Input: part model. Units: mm. Frame: model coordinates. A direction names the side the tool comes from. Give positions to 0.01 mm unless a question says otherwise; leave off trailing zeros. Loops run counter-clockwise (first coordinate to the right, second up) from the corner with the lowest first, then second, coordinate; pieces in that order, holes last. Notation, with made-up numbers: (51.5, 40.5) - (63.5, 40.5) arc R24 ccw to (63.5, 59.5) - close; hole circle Ø9 at (68, 19.25). An arc over 180 degrees is marked (long way). Answer as a JSON object with one key per item and string values.
from build123d import *

# Parameters (mm, degrees)
F0_R     = 3.5
F1_DEPTH = 25
F2_DEPTH = 2
F3_DEPTH = 10
F4_DEPTH = 21


with BuildPart() as f1:
    # F0 (on Top) → F1 (new body)
    with BuildSketch(Plane.XY):
        with BuildLine():
            ThreePointArc((10.25, -7.1545440106), (5, 0), (10.25, 7.1545440106))
            ThreePointArc((10.25, 7.1545440106), (8.8388347648, 8.8388347648), (7.1545440106, 10.25))
            ThreePointArc((7.1545440106, 10.25), (0, 5), (-7.1545440106, 10.25))
            ThreePointArc((-7.1545440106, 10.25), (-8.8388347648, 8.8388347648), (-10.25, 7.1545440106))
            ThreePointArc((-10.25, 7.1545440106), (-6.4533066888, 4.4370598373), (-5, 0))
            ThreePointArc((-5, 0), (-6.4533066888, -4.4370598373), (-10.25, -7.1545440106))
            ThreePointArc((-10.25, -7.1545440106), (-8.8388347648, -8.8388347648), (-7.1545440106, -10.25))
            ThreePointArc((-7.1545440106, -10.25), (0, -5), (7.1545440106, -10.25))
            ThreePointArc((7.1545440106, -10.25), (8.8388347648, -8.8388347648), (10.25, -7.1545440106))
        make_face()
        Circle(F0_R, mode=Mode.SUBTRACT)
        with BuildLine():
            ThreePointArc((-7.1545440106, 10.25), (0, 5), (7.1545440106, 10.25))
            ThreePointArc((7.1545440106, 10.25), (5.3824617408, 11.2818041823), (3.4655302625, 12.01))
            ThreePointArc((3.4655302625, 12.01), (0, 9), (-3.4655302625, 12.01))
            ThreePointArc((-3.4655302625, 12.01), (-5.3824617408, 11.2818041823), (-7.1545440106, 10.25))
        make_face()
        with BuildLine():
            ThreePointArc((-5, 0), (-6.4533066888, 4.4370598373), (-10.25, 7.1545440106))
            ThreePointArc((-10.25, 7.1545440106), (-11.2818041823, 5.3824617408), (-12.01, 3.4655302625))
            ThreePointArc((-12.01, 3.4655302625), (-9.8575579477, 2.2951034835), (-9, 0))
            ThreePointArc((-9, 0), (-9.8575579477, -2.2951034835), (-12.01, -3.4655302625))
            ThreePointArc((-12.01, -3.4655302625), (-11.2818041823, -5.3824617408), (-10.25, -7.1545440106))
            ThreePointArc((-10.25, -7.1545440106), (-6.4533066888, -4.4370598373), (-5, 0))
        make_face()
        with BuildLine():
            ThreePointArc((3.4655302625, -12.01), (5.3824617408, -11.2818041823), (7.1545440106, -10.25))
            ThreePointArc((7.1545440106, -10.25), (0, -5), (-7.1545440106, -10.25))
            ThreePointArc((-7.1545440106, -10.25), (-5.3824617408, -11.2818041823), (-3.4655302625, -12.01))
            ThreePointArc((-3.4655302625, -12.01), (0, -9), (3.4655302625, -12.01))
        make_face()
        with BuildLine():
            ThreePointArc((12.01, -3.4655302625), (9, 0), (12.01, 3.4655302625))
            ThreePointArc((12.01, 3.4655302625), (11.2818041823, 5.3824617408), (10.25, 7.1545440106))
            ThreePointArc((10.25, 7.1545440106), (5, 0), (10.25, -7.1545440106))
            ThreePointArc((10.25, -7.1545440106), (11.2818041823, -5.3824617408), (12.01, -3.4655302625))
        make_face()
        with BuildLine():
            ThreePointArc((10.25, 7.1545440106), (11.2818041823, 5.3824617408), (12.01, 3.4655302625))
            ThreePointArc((12.01, 3.4655302625), (14.7951034835, 2.6424420523), (16, 0))
            ThreePointArc((16, 0), (14.7951034835, -2.6424420523), (12.01, -3.4655302625))
            ThreePointArc((12.01, -3.4655302625), (11.2818041823, -5.3824617408), (10.25, -7.1545440106))
            ThreePointArc((10.25, -7.1545440106), (16.9370598373, -6.0466933112), (20, 0))
            ThreePointArc((20, 0), (16.9370598373, 6.0466933112), (10.25, 7.1545440106))
        make_face()
        with BuildLine():
            ThreePointArc((3.4655302625, 12.01), (5.3824617408, 11.2818041823), (7.1545440106, 10.25))
            ThreePointArc((7.1545440106, 10.25), (7.4131329436, 11.3618172554), (7.5, 12.5))
            ThreePointArc((7.5, 12.5), (-1.1381827446, 19.9131329436), (-7.1545440106, 10.25))
            ThreePointArc((-7.1545440106, 10.25), (-5.3824617408, 11.2818041823), (-3.4655302625, 12.01))
            ThreePointArc((-3.4655302625, 12.01), (-0.2456054574, 15.9913719308), (3.5, 12.5))
            ThreePointArc((3.5, 12.5), (3.4913719308, 12.2543945426), (3.4655302625, 12.01))
        make_face()
    extrude(amount=F1_DEPTH)

    # F0 (on Top) → F2 (join)
    with BuildSketch(Plane.XY):
        with BuildLine():
            ThreePointArc((3.5, -12.5), (3.4913719308, -12.2543945426), (3.4655302625, -12.01))
            ThreePointArc((3.4655302625, -12.01), (2.7345425148, -12.1972241611), (1.9935897271, -12.34))
            ThreePointArc((1.9935897271, -12.34), (1.9983967892, -12.4199358201), (2, -12.5))
            ThreePointArc((2, -12.5), (-0.0800641799, -14.4983967892), (-1.9935897271, -12.34))
            ThreePointArc((-1.9935897271, -12.34), (-2.7345425148, -12.1972241611), (-3.4655302625, -12.01))
            ThreePointArc((-3.4655302625, -12.01), (-0.2456054574, -15.9913719308), (3.5, -12.5))
        make_face()
        with BuildLine():
            ThreePointArc((1.9935897271, -12.34), (2.7345425148, -12.1972241611), (3.4655302625, -12.01))
            ThreePointArc((3.4655302625, -12.01), (0, -9), (-3.4655302625, -12.01))
            ThreePointArc((-3.4655302625, -12.01), (-2.7345425148, -12.1972241611), (-1.9935897271, -12.34))
            ThreePointArc((-1.9935897271, -12.34), (0, -10.5), (1.9935897271, -12.34))
        make_face()
        with BuildLine():
            ThreePointArc((-12.34, 1.9935897271), (-12.1972241611, 2.7345425148), (-12.01, 3.4655302625))
            ThreePointArc((-12.01, 3.4655302625), (-16, 0), (-12.01, -3.4655302625))
            ThreePointArc((-12.01, -3.4655302625), (-12.1972241611, -2.7345425148), (-12.34, -1.9935897271))
            ThreePointArc((-12.34, -1.9935897271), (-14.5, 0), (-12.34, 1.9935897271))
        make_face()
        with BuildLine():
            ThreePointArc((-9, 0), (-9.8575579477, 2.2951034835), (-12.01, 3.4655302625))
            ThreePointArc((-12.01, 3.4655302625), (-12.1972241611, 2.7345425148), (-12.34, 1.9935897271))
            ThreePointArc((-12.34, 1.9935897271), (-11.0303061543, 1.3564659966), (-10.5, 0))
            ThreePointArc((-10.5, 0), (-11.0303061543, -1.3564659966), (-12.34, -1.9935897271))
            ThreePointArc((-12.34, -1.9935897271), (-12.1972241611, -2.7345425148), (-12.01, -3.4655302625))
            ThreePointArc((-12.01, -3.4655302625), (-9.8575579477, -2.2951034835), (-9, 0))
        make_face()
        with BuildLine():
            ThreePointArc((1.9935897271, 12.34), (2.7345425148, 12.1972241611), (3.4655302625, 12.01))
            ThreePointArc((3.4655302625, 12.01), (3.4913719308, 12.2543945426), (3.5, 12.5))
            ThreePointArc((3.5, 12.5), (-0.2456054574, 15.9913719308), (-3.4655302625, 12.01))
            ThreePointArc((-3.4655302625, 12.01), (-2.7345425148, 12.1972241611), (-1.9935897271, 12.34))
            ThreePointArc((-1.9935897271, 12.34), (-0.0800641799, 14.4983967892), (2, 12.5))
            ThreePointArc((2, 12.5), (1.9983967892, 12.4199358201), (1.9935897271, 12.34))
        make_face()
        with BuildLine():
            ThreePointArc((-3.4655302625, 12.01), (0, 9), (3.4655302625, 12.01))
            ThreePointArc((3.4655302625, 12.01), (2.7345425148, 12.1972241611), (1.9935897271, 12.34))
            ThreePointArc((1.9935897271, 12.34), (0, 10.5), (-1.9935897271, 12.34))
            ThreePointArc((-1.9935897271, 12.34), (-2.7345425148, 12.1972241611), (-3.4655302625, 12.01))
        make_face()
        with BuildLine():
            ThreePointArc((12.01, 3.4655302625), (12.1972241611, 2.7345425148), (12.34, 1.9935897271))
            ThreePointArc((12.34, 1.9935897271), (13.8564659966, 1.4696938457), (14.5, 0))
            ThreePointArc((14.5, 0), (13.8564659966, -1.4696938457), (12.34, -1.9935897271))
            ThreePointArc((12.34, -1.9935897271), (12.1972241611, -2.7345425148), (12.01, -3.4655302625))
            ThreePointArc((12.01, -3.4655302625), (14.7951034835, -2.6424420523), (16, 0))
            ThreePointArc((16, 0), (14.7951034835, 2.6424420523), (12.01, 3.4655302625))
        make_face()
        with BuildLine():
            ThreePointArc((12.34, -1.9935897271), (10.5, 0), (12.34, 1.9935897271))
            ThreePointArc((12.34, 1.9935897271), (12.1972241611, 2.7345425148), (12.01, 3.4655302625))
            ThreePointArc((12.01, 3.4655302625), (9, 0), (12.01, -3.4655302625))
            ThreePointArc((12.01, -3.4655302625), (12.1972241611, -2.7345425148), (12.34, -1.9935897271))
        make_face()
    extrude(amount=F2_DEPTH)

    # F0 (on Top) → F3 (join)
    with BuildSketch(Plane.XY):
        with BuildLine():
            ThreePointArc((-12.01, 3.4655302625), (-11.2818041823, 5.3824617408), (-10.25, 7.1545440106))
            ThreePointArc((-10.25, 7.1545440106), (-20, 0), (-10.25, -7.1545440106))
            ThreePointArc((-10.25, -7.1545440106), (-11.2818041823, -5.3824617408), (-12.01, -3.4655302625))
            ThreePointArc((-12.01, -3.4655302625), (-16, 0), (-12.01, 3.4655302625))
        make_face()
        with BuildLine():
            ThreePointArc((7.5, -12.5), (7.4131329436, -11.3618172554), (7.1545440106, -10.25))
            ThreePointArc((7.1545440106, -10.25), (5.3824617408, -11.2818041823), (3.4655302625, -12.01))
            ThreePointArc((3.4655302625, -12.01), (3.4913719308, -12.2543945426), (3.5, -12.5))
            ThreePointArc((3.5, -12.5), (-0.2456054574, -15.9913719308), (-3.4655302625, -12.01))
            ThreePointArc((-3.4655302625, -12.01), (-5.3824617408, -11.2818041823), (-7.1545440106, -10.25))
            ThreePointArc((-7.1545440106, -10.25), (-1.1381827446, -19.9131329436), (7.5, -12.5))
        make_face()
    extrude(amount=F3_DEPTH)

    # F0 (on Top) → F4 (join)
    with BuildSketch(Plane.XY):
        Circle(F0_R)
    extrude(amount=F4_DEPTH)


solid = f1.part
Item 1: Cut plane B-B (y = 13). Return loops of the section in (x, z).
Geometry check:
{"outline": "(-7.48, 0) - (-1.94, 0) - (-1.94, 2) - (-3.46, 2) - (-3.46, 25) - (-7.48, 25) - close; (1.94, 0) - (7.48, 0) - (7.48, 25) - (3.46, 25) - (3.46, 2) - (1.94, 2) - close"}
Item 2: Cut plane C-C (z = 6.75). Return loops of the section in (x, y), then the cut area to 3 significant figures.
Geometry check:
{"outline": "(-10.25, -7.15) arc R12.5 ccw to (-7.15, -10.25) arc R7.5 ccw (long way) to (7.15, -10.25) arc R12.5 ccw to (10.25, -7.15) arc R7.5 ccw (long way) to (10.25, 7.15) arc R12.5 ccw to (7.15, 10.25) arc R7.5 ccw (long way) to (-7.15, 10.25) arc R12.5 ccw to (-10.25, 7.15) arc R7.5 ccw (long way) to start; hole circle Ø7 at (-12.5, 0); hole circle Ø7 at (0, -12.5); hole circle Ø7 at (0, 12.5); hole circle Ø7 at (12.5, 0)", "area": "736 mm2"}
Item 3: Cut plane D-D (x = -6). Return loops of the section in (y, z).
Geometry check:
{"outline": "(-17, 0) - (17, 0) - (17, 25) - (-10.97, 25) - (-10.97, 10) - (-17, 10) - close"}
Item 4: Contact query for flat-ended pins moving along their axis: P1, Ø2, axis at x = -11, y = 1, coming from the +Z side; P2, Ø2.5, axis at x = -12.5, y = 0, coming from the -Z side; P3, Ø4, axis at x = -5.5, y = -7.5, coming from the -Z side; P4, Ø10.5, axis at x = -2, y = -17.5, coming from the +Z side. Output: stop coordinate, or through.
Geometry check:
{"P1": "stops at z = 2", "P2": "passes through", "P3": "stops at z = 0", "P4": "stops at z = 10"}
Item 5: Access query for faces 3 (the face through (3.233, -1.341, 22.972)), 4 (the face through (-20, 0, 5)). Directions: +Z, -Z, +X, -X, +Y, -Y. A direction counts if a zero-diameter tool reaches every point of the face in a straight line with its end or side. Return the directions, or none.
Geometry check:
{"face 3": "+Z", "face 4": "+Z, -Z"}
Item 6: Mould query, pull axis X, two halves, no side actions, for faces 1 (the face through (-16.3, 0.1, 10)), 2 (the face through (-11, -2, 2)). Classes: released by +X, released by -X, zero draft, split by the parting line, or undercut.
Geometry check:
{"face 1": "zero draft", "face 2": "undercut"}
Item 7: Material intervals for line 1 (Y direction, x = 0, z = 22.75); line 2 (Y direction, x = 0, z = 5.5); line 3 (Y direction, x = -12.5, z = 5.5), sorted ascending. Write a range as [from, to].
Geometry check:
{"line 1": "y = [-9, -3.5], [3.5, 9], [16, 20]", "line 2": "y = [-20, -16], [-9, 9], [16, 20]", "line 3": "y = [-7.5, -3.5], [3.5, 7.5]"}
Item 8: Cut plane A-A (x = 0). Return loops of the section in (y, z).
Geometry check:
{"outline": "(-20, 0) - (-14.5, 0) - (-14.5, 2) - (-16, 2) - (-16, 10) - (-20, 10) - close; (-10.5, 0) - (10.5, 0) - (10.5, 2) - (9, 2) - (9, 25) - (3.5, 25) - (3.5, 21) - (-3.5, 21) - (-3.5, 25) - (-9, 25) - (-9, 2) - (-10.5, 2) - close; (14.5, 0) - (20, 0) - (20, 25) - (16, 25) - (16, 2) - (14.5, 2) - close"}
